Design review of the part built by this model. Coordinates are the model's own, in mm. Face numbers are marked on the shaded views. A direction names the side the tool comes from. Give positions to 0.01 mm unless a question says otherwise; leave off trailing zeros. Loops run counter-clockwise (first coordinate to the right, second up) from the corner with the lowest first, then second, coordinate; pieces in that order, holes last. Notation, with made-up numbers: (36.25, -23.5) -> (69.25, -23.5) arc R30 ccw to (69.25, 8.5) -> close; hole circle Ø10 at (88, -18). An arc over 180 degrees is marked (long way). Use CSV: the item, a comma, the result in double quotes. Start each with the question number.
Item 1: Clearance check with flat-ended pins moving along their axes: pin 1 (12 mm diameter, centred on x = 85, z = -148, fed in from -Y); pin 2 (6 mm diameter, centred on x = -40, z = -86, fed in from -Y); pin 3 (10 mm diameter, centred on y = -49.5, z = -487.5, fed in from -X). State where each tip first meets the part, or that it passes through.
Item 2: The part is to be moulded in two halves that separate along X. For the marked faces 1, 2 and 3, say which applies: +X half, -X half, draft (parallel to the pull), parting line (faces both ways), or undercut.
Item 3: For the marked faces 4, 5 and 6, list the 3-axis set-ups (+Z, -Z, +X, -X, +Y, -Y) from which the entire face can be reached by the end or side of a thin tool; tool diameter is ignored.
Item 4: We need section B-B (z = -433.5). State the section outline as (x, y) points, plus the area to 3 significant figures.
Item 5: Wall thickness on line 1 along Y through (x, z) = (0, -306.5); line 2 along Y through (x, z) = (0, -143); line 3 along Z through (x, y) = (-157.5, -39.5): over which ranges is each line inside the solid? List them lowest first. Write a range as from..to.
Item 6: We need section A-A (z = -187.5). State the section outline as (x, y) points, plus the area to 3 significant figures.
from build123d import *

# Parameters (mm, degrees)
BOSS_EXTRUDE1_DEPTH = 10
SKETCH5_R           = 180
SKETCH5_R_2         = 90.447985836
BOSS_EXTRUDE2_DEPTH = 84
CHAMFER1_SIZE       = 50


with BuildPart() as part:
    # Sketch2 → Revolve1 (revolve)
    with BuildSketch(Plane(origin=(0, 0, 0), x_dir=(0, 0, -1), z_dir=(1, 0, 0)), mode=Mode.PRIVATE) as revolve1_sk:
        with BuildLine():
            Line((0, 0), (700, 0))
            Line((700, 0), (720, 0))
            ThreePointArc((720, 0), (714.142135624, 14.142135624), (700, 20))
            Line((700, 20), (575.510554629, 35.889479609))
            Line((575.510554629, 35.889479609), (545.741946393, 35.889479609))
            Line((545.741946393, 35.889479609), (545.741946393, 24))
            Line((545.741946393, 24), (492, 24))
            Line((492, 24), (492, 92.350959719))
            Line((492, 92.350959719), (270.736708403, 92.350959719))
            Line((270.736708403, 92.350959719), (180, 118.736948211))
            Line((180, 118.736948211), (0, 118.736948211))
            Line((0, 118.736948211), (0, 0))
        make_face()
    revolve(revolve1_sk.sketch.rotate(Axis((0, 0, 0), (0, 0, -1)), 90), axis=Axis((0, 0, 0), (0, 0, -1)))

    # Sketch3 → Boss-Extrude1 (add)
    with BuildSketch(Plane.XY.offset(-545.741946393)):
        Polygon((47.46164508, -5.94638242), (28.880540777, 38.129799135), (-18.581104304, 44.076181555), (-47.46164508, 5.94638242), (-28.880540777, -38.129799135), (18.581104304, -44.076181555), align=None)
    extrude(amount=BOSS_EXTRUDE1_DEPTH)

    # Sketch4 → Cut-Revolve6 (revolve, cut)
    with BuildSketch(Plane(origin=(0, 0, 0), x_dir=(0, 0, -1), z_dir=(1, 0, 0)), mode=Mode.PRIVATE) as cut_revolve6_sk:
        Polygon((0, 0), (720, 0), (720, 4.24350933), (575.510554629, 16.375367187), (477.848045129, 16.375367187), (416.651810859, 69.245469072), (270.736708403, 69.245469072), (179.731042443, 90.447985836), (0, 90.447985836), align=None)
    revolve(cut_revolve6_sk.sketch.rotate(Axis((0, 0, 0), (0, 0, -1)), 90), axis=Axis((0, 0, 0), (0, 0, -1)), mode=Mode.SUBTRACT)

    # Sketch5 → Boss-Extrude2 (add)
    with BuildSketch(Plane.XY):
        Circle(SKETCH5_R)
        Circle(SKETCH5_R_2, mode=Mode.SUBTRACT)
    extrude(amount=-BOSS_EXTRUDE2_DEPTH)

    # Chamfer1
    chamfer1_edges = [part.edges().sort_by_distance(p)[0] for p in [
        (-118.736948211, 0, -84),
    ]]
    chamfer(chamfer1_edges, length=CHAMFER1_SIZE)


solid = part.part
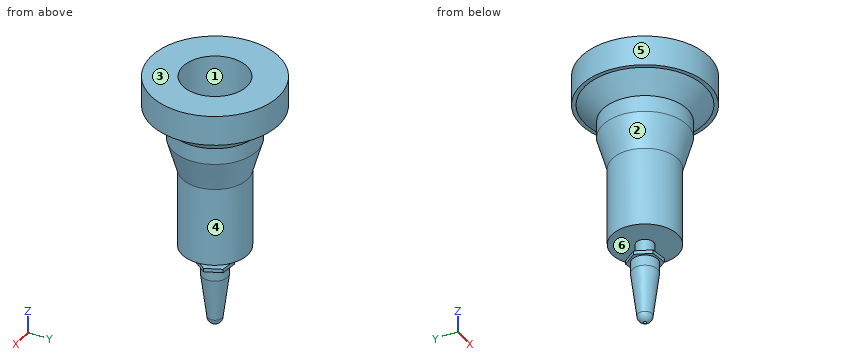
Results found:
1,pin 1,"y = -88.64"
1,pin 2,"y = -175.99"
1,pin 3,"x = -80.92"
2,face 1,"undercut"
2,face 2,"parting line"
2,face 3,"draft"
3,face 4,"-Z"
3,face 5,"+Z, -Z"
3,face 6,"none"
4,outline,"circle Ø184.7 at (0, 0); hole circle Ø109.38 at (0, 0)"
4,area,"17,400 mm²"
5,line 1,"-92.35..-69.25, 69.25..92.35"
5,line 2,"-118.74..-90.45, 90.45..118.74"
5,line 3,"-90.36..0"
6,outline,"circle Ø233.11 at (0, 0); hole circle Ø177.28 at (0, 0)"
6,area,"18,000 mm²"
